from build123d import *

# Parameters (mm, degrees)
F0_R     = 8.5
F0_R_2   = 7.5
F1_ANGLE = 90
F2_R     = 9
F2_R_2   = 7.25
F3_DEPTH = 12.5
F4_R     = 9
F4_R_2   = 7.25
F5_DEPTH = 12.5


# Not quite as in the source:
# - a fillet or chamfer that OpenCascade refuses, or shapes differently, is made with other operations: its cross-section is extruded or revolved along the edge and cut away or added


with BuildPart() as f1:
    # F0 (on Front) → F1 (revolve)
    with BuildSketch(Plane.XZ):
        Circle(F0_R)
        Circle(F0_R_2, mode=Mode.SUBTRACT)
    revolve(axis=Axis((-10, 0, 0.1811354887), (0, 0, -1)), revolution_arc=F1_ANGLE)

    # F2 (on Front) → F3 (join)
    with BuildSketch(Plane.XZ):
        Circle(F2_R)
        Circle(F2_R_2, mode=Mode.SUBTRACT)
    extrude(amount=-F3_DEPTH)

    # F4 (on face) → F5 (join)
    with BuildSketch(Plane(origin=(-10, 0, 0), x_dir=(0, -1, 0), z_dir=(-1, 0, 0))):
        with Locations((10, 0)):
            Circle(F4_R)
        with Locations((10, 0)):
            Circle(F4_R_2, mode=Mode.SUBTRACT)
    extrude(amount=F5_DEPTH)

    # F6: fillet of radius 5 on 2 edges, made by hand

    # F6_s1 → F6_t2 (revolve, cut)
    with BuildSketch(Plane.XY):
        with BuildLine():
            ThreePointArc((-12.1794494718, -19), (-11.061415483, -18.8733971724), (-10, -18.5))
            Line((-10, -18.5), (-10, -19))
            Line((-10, -19), (-12.1794494718, -19))
        make_face()
    revolve(axis=Axis((-10, -10, 0), (-1, 0, 0)), mode=Mode.SUBTRACT)

    # F6_s3 → F6_t4 (revolve, cut)
    with BuildSketch(Plane.XY):
        with BuildLine():
            ThreePointArc((8.5, 0), (8.8733971724, 1.061415483), (9, 2.1794494718))
            Line((9, 2.1794494718), (9, 0))
            Line((9, 0), (8.5, 0))
        make_face()
    revolve(axis=Axis((0, 0, 0), (0, -1, 0)), mode=Mode.SUBTRACT)


solid = f1.part
Model file for the job. Use its own axes, mm. A direction names the side the tool comes from. Coordinates: 2 decimals unless noted, no trailing zeros. Loops run counter-clockwise (first coordinate to the right, second up) from the corner with the lowest first, then second, coordinate; pieces in that order, holes last. Notation, with made-up numbers: (-1.75, -24) -> (7.25, -24) arc R15 ccw to (7.25, -18) -> close; hole circle Ø8 at (24.25, -33). An arc over 180 degrees is marked (long way). Use one line per item in the form item = value. Start each with the question number.
(1) Flat gauge pins, fed straight in: pin 1 (5 mm diameter, centred on x = -4, y = -5, fed in from +Z); pin 2 (2 mm diameter, centred on y = 8, z = 2, fed in from -X); pin 3 (2 mm diameter, centred on x = 3.5, y = -3.5, fed in from +Z). Where does each tip first touch, or does it go through?
(2) Pull direction X, two halves, no side cores. Call faces 1 (the flat face through (-22.5, -10.6, 7.4)), 2 (the cylindrical face through (-16.163, -4.247, -4.412)), 3 (the cylindrical face through (3.35, 6.16, -6.43)), 4 (the cylindrical face through (-1.172, 7.267, 8.923)): pulls with the +X half, pulls with the -X half, needs draft (parallel to the pull), parting line crosses it, or undercut.
(3) Cut at A-A on x = -18. Give the cut face in (y, z).
(4) Probe probe 1 along Z at (x, y) = (-18, -10); probe 2 along X at (y, z) = (-4.5, -6); probe 3 along Z at (x, y) = (-5, -14). List the from-to ranges inside material, lowest first. Write a range as from..to.
(5) Tool access for faces 5 (the flat face through (0.6, 12.5, 7.4)), 6 (the cylindrical face through (-17.267, -18.584, 2.703)): list every direction of +Z, -Z, +X, -X, +Y, -Y with a clear straight run to the whole face (end or side of a thin tool).
Values:
q1.pin_1 = 8.5
q1.pin_2 = -8.94
q1.pin_3 = 7.97
q2.face_1 = pulls with the -X half
q2.face_2 = needs draft
q2.face_3 = undercut
q2.face_4 = parting line crosses it
q3.outline = circle Ø18 at (-10, 0); hole circle Ø14.5 at (-10, 0)
q4.probe_1 = -9..-7.25, 7.25..9
q4.probe_2 = -22.5..-6.84, 3.78..5.38
q4.probe_3 = -6.97..-5.71, 5.71..6.97
q5.face_5 = +Z, -Z, +X, -X, +Y
q5.face_6 = -X
